```python
from build123d import *
from build123d.topology import SkipClean

# Parameters (mm, degrees)
CROQUIS3_W              = 38
CROQUIS3_H              = 23
CROQUIS3_R              = 1.75
SALIENTE_EXTRUIR1_DEPTH = 1
SALIENTE_EXTRUIR2_DEPTH = 25
SALIENTE_EXTRUIR4_DEPTH = 40
SALIENTE_EXTRUIR5_DEPTH = 6
CORTAR_EXTRUIR3_DEPTH   = 65.46296637
CROQUIS5_R              = 1.75
CORTAR_EXTRUIR1_DEPTH   = 12
CROQUIS11_R             = 1.75
CORTAR_EXTRUIR4_DEPTH   = 58.245149126
CORTAR_EXTRUIR5_DEPTH   = 58.134007224
REDONDEO1_R             = 2
SALIENTE_EXTRUIR6_START = 2
CROQUIS13_R             = 1.75
SALIENTE_EXTRUIR6_DEPTH = 2
CHAFL_N1_SIZE           = 1
CORTAR_EXTRUIR6_DEPTH   = 64.102925108
SALIENTE_EXTRUIR7_DEPTH = 3


with BuildPart() as part:
    # Croquis3 → Saliente-Extruir1 (new body)
    with BuildSketch(Plane.XY.offset(-3)):
        with Locations((22, 0)):
            Rectangle(CROQUIS3_W, CROQUIS3_H)
        with Locations((9.5, 8.75)):
            Circle(CROQUIS3_R, mode=Mode.SUBTRACT)
        with Locations((9.5, -8.75)):
            Circle(CROQUIS3_R, mode=Mode.SUBTRACT)
        with BuildLine():
            ThreePointArc((20.184659091, -1.912872928), (40, 0), (20.184659091, 1.912872928))
            ThreePointArc((20.184659091, 1.912872928), (16.75, 0), (20.184659091, -1.912872928))
        make_face(mode=Mode.SUBTRACT)
    extrude(amount=SALIENTE_EXTRUIR1_DEPTH)

    # Croquis4 → Saliente-Extruir2 (add)
    with BuildSketch(Plane(origin=(3, 0, 0), x_dir=(0, 0, -1), z_dir=(1, 0, 0))):
        with BuildLine():
            Line((3, 1), (3, -1))
            ThreePointArc((3, -1), (0, -4), (-3, -1))
            Line((-3, -1), (-3, 1))
            ThreePointArc((-3, 1), (0, 4), (3, 1))
        make_face()
    extrude(amount=SALIENTE_EXTRUIR2_DEPTH)



with BuildPart() as body_2:
    # Croquis8 → Saliente-Extruir4 (new body)
    with BuildSketch(Plane(origin=(49, 0, 0), x_dir=(0.8746197071393935, 0.48480962024634133, 0), z_dir=(-0.48480962024634133, 0.8746197071393935, 0))):
        with BuildLine():
            Line((-1, 3), (1, 3))
            ThreePointArc((1, 3), (4, 0), (1, -3))
            Line((1, -3), (-1, -3))
            ThreePointArc((-1, -3), (-4, 0), (-1, 3))
        make_face()
    extrude(amount=SALIENTE_EXTRUIR4_DEPTH)


with BuildPart() as part_1:
    add(part.part)

    add(body_2.part)  # Saliente-Extruir5 merges body 2
    # Croquis9 → Saliente-Extruir5 (add)
    with BuildSketch(Plane.XY.offset(-3)):
        with BuildLine():
            Line((25.151903798, 8.746197071), (39.686136808, 16.802653985))
            Line((39.686136808, 16.802653985), (36.292469466, 22.924991935))
            Line((36.292469466, 22.924991935), (21.758236456, 14.868535021))
            ThreePointArc((21.758236456, 14.868535021), (15.352304272, 8.62815217), (13, 0))
            Line((13, 0), (20, 0))
            ThreePointArc((20, 0), (21.383708396, 5.07538363), (25.151903798, 8.746197071))
        make_face()
    extrude(amount=SALIENTE_EXTRUIR5_DEPTH)

    # Croquis10 → Cortar-Extruir3 (cut, through all)
    with BuildSketch(Plane(origin=(0, 0, -3), x_dir=(-1, 0, 0), z_dir=(0, 0, -1))):
        with BuildLine():
            Line((-54.752227431, 25.153924387), (-25.151903798, 8.746197071))
            ThreePointArc((-25.151903798, 8.746197071), (-21.926969684, 5.901371155), (-20.195, 1.96519083))
            ThreePointArc((-20.195, 1.96519083), (-16.702679258, 0.110983813), (-20, -2.071231518))
            Line((-20, -2.071231518), (-20, -15.393420546))
            Line((-20, -15.393420546), (-54.752227431, -15.393420546))
            Line((-54.752227431, -15.393420546), (-54.752227431, 25.153924387))
        make_face()
    extrude(amount=-CORTAR_EXTRUIR3_DEPTH, mode=Mode.SUBTRACT)

    # Croquis5 → Cortar-Extruir1 (cut)
    with BuildSketch(Plane(origin=(3, 0, 0), x_dir=(0, 0, -1), z_dir=(1, 0, 0))):
        Circle(CROQUIS5_R)
    extrude(amount=CORTAR_EXTRUIR1_DEPTH, mode=Mode.SUBTRACT)

    # Croquis11 → Cortar-Extruir4 (cut, through all)
    with BuildSketch(Plane(origin=(-7.875406784, 14.20760993, 0), x_dir=(0.8746197071393934, 0.4848096202463414, 0), z_dir=(-0.48480962024634144, 0.8746197071393935, 0))):
        with Locations(Location((42.85636565, 0, 0), (0, 0, 180))):
            Circle(CROQUIS11_R)
    extrude(amount=-CORTAR_EXTRUIR4_DEPTH, mode=Mode.SUBTRACT)

    # Croquis12 → Cortar-Extruir5 (cut, through all)
    with BuildSketch(Plane(origin=(0, 0, -3), x_dir=(-1, 0, 0), z_dir=(0, 0, -1))):
        Polygon((-41.818249172, 31.029855201), (-23.89343012, 27.219817295), (-26.84914243, 44.519393877), align=None)
    extrude(amount=-CORTAR_EXTRUIR5_DEPTH, mode=Mode.SUBTRACT)

    # Redondeo1
    redondeo1_edges = [part_1.edges().sort_by_distance(p)[0] for p in [
        (20, -11.5, -2.5),
        (3, 11.5, -2.5),
        (3, -11.5, -2.5),
    ]]
    fillet(redondeo1_edges, radius=REDONDEO1_R)

    # Croquis13 → Saliente-Extruir6 (add)
    with SkipClean():  # the faces are left unmerged after this step: merging them gives an invalid solid
        with BuildSketch(Plane(origin=(0, 0, -3), x_dir=(-1, 0, 0), z_dir=(0, 0, -1)).offset(SALIENTE_EXTRUIR6_START)):
            with BuildLine():
                Line((-20, -2.071231518), (-20, -9.5))
                ThreePointArc((-20, -9.5), (-19.414213562, -10.914213562), (-18, -11.5))
                Line((-18, -11.5), (-5, -11.5))
                ThreePointArc((-5, -11.5), (-3.585786438, -10.914213562), (-3, -9.5))
                Line((-3, -9.5), (-3, 9.5))
                ThreePointArc((-3, 9.5), (-3.585786438, 10.914213562), (-5, 11.5))
                Line((-5, 11.5), (-17.480015974, 11.5))
                ThreePointArc((-17.480015974, 11.5), (-19.483379935, 13.35667258), (-21.758236456, 14.868535021))
                Line((-21.758236456, 14.868535021), (-35.417849759, 22.440182315))
                Line((-35.417849759, 22.440182315), (-31.832998763, 28.907424707))
                Line((-31.832998763, 28.907424707), (-33.878680529, 29.342247789))
                Line((-33.878680529, 29.342247789), (-40.560756515, 17.287463605))
                Line((-40.560756515, 17.287463605), (-25.151903798, 8.746197071))
                ThreePointArc((-25.151903798, 8.746197071), (-21.926969684, 5.901371155), (-20.195, 1.96519083))
                ThreePointArc((-20.195, 1.96519083), (-16.702679258, 0.110983813), (-20, -2.071231518))
            make_face()
            with Locations((-9.5, -8.75)):
                Circle(CROQUIS13_R, mode=Mode.SUBTRACT)
            with Locations((-9.5, 8.75)):
                Circle(CROQUIS13_R, mode=Mode.SUBTRACT)
        extrude(amount=-SALIENTE_EXTRUIR6_DEPTH)

    # Chaflán1
    chafl_n1_edges = [part_1.edges().sort_by_distance(p)[0] for p in [
        (7.75, 8.75, -2),
        (7.75, -8.75, -2),
    ]]
    chamfer(chafl_n1_edges, length=CHAFL_N1_SIZE - 0.0001)  # a hair under: the kernel refuses the full size

    # Croquis14 → Cortar-Extruir6 (cut, through all)
    with BuildSketch(Plane(origin=(3, 0.024746159, -35.327414791), x_dir=(0, 0, 1), z_dir=(-1, 0, 0))):
        with BuildLine():
            ThreePointArc((-38.672585209, 3.211321818), (-41.89733008, 3.713866628), (-43.672585209, 0.975253841))
            Line((-43.672585209, 0.975253841), (-43.672585209, 29.969736253))
            Line((-43.672585209, 29.969736253), (-35.672585209, 29.969736253))
            Line((-35.672585209, 29.969736253), (-35.672585209, 11.475253841))
            Line((-35.672585209, 11.475253841), (-38.672585209, 11.475253841))
            Line((-38.672585209, 11.475253841), (-38.672585209, 3.211321818))
        make_face()
        with BuildLine():
            Line((30.327414791, 11.475253841), (33.327414791, 11.475253841))
            Line((33.327414791, 11.475253841), (33.327414791, 9.475253841))
            Line((33.327414791, 9.475253841), (33.327414791, 3.211321818))
            ThreePointArc((33.327414791, 3.211321818), (36.552159663, 3.713866628), (38.327414791, 0.975253841))
            Line((38.327414791, 0.975253841), (38.327414791, 29.969736253))
            Line((38.327414791, 29.969736253), (30.327414791, 29.969736253))
            Line((30.327414791, 29.969736253), (30.327414791, 11.475253841))
        make_face()
    extrude(amount=-CORTAR_EXTRUIR6_DEPTH, mode=Mode.SUBTRACT)

    # Croquis15 → Saliente-Extruir7 (add)
    with BuildSketch(Plane.XY.offset(-2)):
        with BuildLine():
            Line((3, 9.5), (3, 11.5))
            Line((3, 11.5), (5, 11.5))
            ThreePointArc((5, 11.5), (3.585786438, 10.914213562), (3, 9.5))
        make_face()
    extrude(amount=-SALIENTE_EXTRUIR7_DEPTH)


solid = part_1.part
```
Input: part model. Units: mm. Frame: model coordinates. A direction names the side the tool comes from. Round coordinates to 2 decimals unless told otherwise and drop trailing zeros. Loops run counter-clockwise (first coordinate to the right, second up) from the corner with the lowest first, then second, coordinate; pieces in that order, holes last. Notation, with made-up numbers: (46.25, -10) -> (105.25, -10) arc R36 ccw to (105.25, 28) -> close; hole circle Ø2 at (69.25, -22). An arc over 180 degrees is marked (long way). One line per item, written item: value.
(1) Pin query (flat end, axial travel): pin 1 (4 mm diameter, centred on x = 12, y = 7, fed in from +Z); pin 2 (3 mm diameter, centred on x = 15.5, z = 2, fed in from -Y); pin 3 (3 mm diameter, centred on y = 0, z = 0, fed in from +X). Return the tip coordinate at first contact, or that it passes through.
Geometry check:
pin 1: z = -2
pin 2: y = -3.96
pin 3: x = 17.26
(2) Section D-D (y = 0). Return the cut outline in (x, z), plus the area to 3 significant figures.
Geometry check:
outline: (3, -5) -> (16.7, -5) -> (16.7, 3) -> (3, 3) -> (3, 1.75) -> (15, 1.75) -> (15, -1.75) -> (3, -1.75) -> close
area: 67.6 mm2
(3) Set-up query: faces 1 (the face through (11, -11.5, -4)), 2 (the face through (8.916, -0.67, -1.617)), 3 (the face through (20, -5, -3)). Return all of +Z, -Z, +X, -X, +Y, -Y with unobstructed straight access to the full face (end or side cutting, diameter ignored); none if empty.
Geometry check:
face 1: +Z, -Z, +X, -X, -Y
face 2: -X
face 3: +Z, -Z, +X, -Y
(4) Mould query, pull axis Z, two halves, no side actions, for faces 4 (the face through (14, 0, -5)), 5 (the face through (16.707, 0.177, -1.056)), 6 (the face through (15, 0, 0)). Classes: pulls with the +Z half, pulls with the -Z half, needs draft (parallel to the pull), parting line crosses it, or undercut.
Geometry check:
face 4: pulls with the -Z half
face 5: needs draft
face 6: undercut
